from build123d import *
from build123d.topology import SkipClean

# Parameters (mm, degrees)
ESQUISSE2_R                                      = 31.5
ESQUISSE2_W                                      = 32
ESQUISSE2_H                                      = 32
BOSS_EXTRU_1_DEPTH                               = 3
BOSS_EXTRU_2_START                               = -100
ESQUISSE4_R                                      = 35
ESQUISSE4_R_2                                    = 31.5
BOSS_EXTRU_2_DEPTH                               = 100
BOSS_EXTRU_3_OUTLINE_R                           = 31.5
BOSS_EXTRU_3_OUTLINE_W                           = 43
BOSS_EXTRU_3_OUTLINE_H                           = 42.5
BOSS_EXTRU_3_DEPTH                               = 97
ESQUISSE6_R                                      = 31.5
ENL_V_MAT_EXTRU_1_DEPTH                          = 10
ESQUISSE7_R                                      = 49
ESQUISSE7_R_2                                    = 35
BOSS_EXTRU_4_DEPTH                               = 10
BOSS_EXTRU_5_START                               = 30
BOSS_EXTRU_5_DEPTH                               = 30
BOSS_EXTRU_6_START                               = 16
BOSS_EXTRU_6_DEPTH                               = 16
CONG_1_R                                         = 10
ESQUISSE11_W                                     = 137.068824
ESQUISSE11_H                                     = 50.889867
ENL_V_MAT_EXTRU_2_DEPTH                          = 153
CHAMBRAGE_POUR_VIS_T_TE_RONDE_6_PANS_D           = 5.3
CHAMBRAGE_POUR_VIS_T_TE_RONDE_6_PANS_DEPTH       = 18
CHAMBRAGE_POUR_VIS_T_TE_RONDE_6_PANS_CBORE_D     = 10.5
CHAMBRAGE_POUR_VIS_T_TE_RONDE_6_PANS_CBORE_DEPTH = 2.75
CHAMBRAGE_POUR_VIS_T_TE_RONDE_6_PANS_TIP         = 1.592281
ESQUISSE18_R                                     = 2.6
ENL_V_MAT_EXTRU_4_DEPTH                          = 25
ESQUISSE19_R                                     = 4.6
ENL_V_MAT_EXTRU_5_DEPTH                          = 25
ESQUISSE20_W                                     = 2
ESQUISSE20_H                                     = 3
ENL_V_MAT_EXTRU_6_DEPTH                          = 45
ENL_V_START                                      = -90
ENL_V_MAT_EXTRU_7_DEPTH                          = 90


# Read off the part's stored shape, not the designer's step: Boss.-Extru.3
with BuildPart() as part:
    # Esquisse2 → Boss.-Extru.1 (new body)
    with BuildSketch(Plane.XY):
        Circle(ESQUISSE2_R)
        with Locations((0.409228, -1.432297)):
            Rectangle(ESQUISSE2_W, ESQUISSE2_H, mode=Mode.SUBTRACT)
    extrude(amount=BOSS_EXTRU_1_DEPTH)

    # Esquisse4 → Boss.-Extru.2 (add)
    with BuildSketch(Plane.XY.offset(3).offset(BOSS_EXTRU_2_START)):
        Circle(ESQUISSE4_R)
        Circle(ESQUISSE4_R_2, mode=Mode.SUBTRACT)
    extrude(amount=BOSS_EXTRU_2_DEPTH)

    # Boss.-Extru.3 outline → Boss.-Extru.3 (add)
    with BuildSketch(Plane(origin=(0, 0, 0), x_dir=(-1, 0, 0), z_dir=(0, 0, -1))):
        Circle(BOSS_EXTRU_3_OUTLINE_R)
        with Locations((-0.409228, -1.182297)):
            Rectangle(BOSS_EXTRU_3_OUTLINE_W, BOSS_EXTRU_3_OUTLINE_H, mode=Mode.SUBTRACT)
    extrude(amount=BOSS_EXTRU_3_DEPTH)

    # Esquisse6 → Enlèv. mat.-Extru.1 (cut)
    with BuildSketch(Plane(origin=(0, 0, -97), x_dir=(-1, 0, 0), z_dir=(0, 0, -1))):
        Circle(ESQUISSE6_R)
    extrude(amount=-ENL_V_MAT_EXTRU_1_DEPTH, mode=Mode.SUBTRACT)

    # Esquisse7 → Boss.-Extru.4 (add)
    with BuildSketch(Plane(origin=(0, 0, -97), x_dir=(-1, 0, 0), z_dir=(0, 0, -1))):
        Circle(ESQUISSE7_R)
        with Locations(Location((0, 0, 0), (0, 0, 180))):
            Circle(ESQUISSE7_R_2, mode=Mode.SUBTRACT)
    extrude(amount=-BOSS_EXTRU_4_DEPTH)

    # Esquisse8 → Boss.-Extru.5 (add)
    with SkipClean():  # the faces are left unmerged after this step: merging them gives an invalid solid
        with BuildSketch(Plane(origin=(0, 0, -97), x_dir=(-1, 0, 0), z_dir=(0, 0, -1)).offset(BOSS_EXTRU_5_START)):
            with BuildLine():
                Line((-47.96874, 10), (-29.870554, 10))
                ThreePointArc((-29.870554, 10), (-31.5, 0), (-29.870554, -10))
                Line((-29.870554, -10), (-47.96874, -10))
                ThreePointArc((-47.96874, -10), (-49, 0), (-47.96874, 10))
            make_face()
            with BuildLine():
                Line((29.870554, 10), (47.96874, 10))
                ThreePointArc((47.96874, 10), (49, 0), (47.96874, -10))
                Line((47.96874, -10), (29.870554, -10))
                ThreePointArc((29.870554, -10), (31.5, 0), (29.870554, 10))
            make_face()
        extrude(amount=-BOSS_EXTRU_5_DEPTH)

    # Esquisse10 → Boss.-Extru.6 (add)
    with SkipClean():  # the faces are left unmerged after this step: merging them gives an invalid solid
        with BuildSketch(Plane(origin=(0, 0, -127), x_dir=(-1, 0, 0), z_dir=(0, 0, -1)).offset(BOSS_EXTRU_6_START)):
            with BuildLine():
                Line((47.96874, 10), (-47.96874, 10))
                ThreePointArc((-47.96874, 10), (-49, 0), (-47.96874, -10))
                Line((-47.96874, -10), (47.96874, -10))
                ThreePointArc((47.96874, -10), (49, 0), (47.96874, 10))
            make_face()
        extrude(amount=-BOSS_EXTRU_6_DEPTH)

    # Congé1
    cong_1_edges = [part.edges().sort_by_distance(p)[0] for p in [
        (-49, 0, -143),
        (49, 0, -143),
    ]]
    fillet(cong_1_edges, radius=CONG_1_R)

    # Esquisse11 → Enlèv. mat.-Extru.2 (cut)
    with SkipClean():  # the faces are left unmerged after this step: merging them gives an invalid solid
        with BuildSketch(Plane(origin=(0, 0, -143), x_dir=(-1, 0, 0), z_dir=(0, 0, -1))):
            with Locations((0, -25.444933)):
                Rectangle(ESQUISSE11_W, ESQUISSE11_H)
        extrude(amount=-ENL_V_MAT_EXTRU_2_DEPTH, mode=Mode.SUBTRACT)

    # Chambrage pour Vis à tête ronde à 6 pans creux M51
    with Locations(Plane(origin=(0, 10, 0), x_dir=(1, 0, 0), z_dir=(0, 1, 0))):
        with Locations((-38.919647, 112), (38.919647, 112), (0, 135)):
            CounterBoreHole(CHAMBRAGE_POUR_VIS_T_TE_RONDE_6_PANS_D / 2, CHAMBRAGE_POUR_VIS_T_TE_RONDE_6_PANS_CBORE_D / 2, CHAMBRAGE_POUR_VIS_T_TE_RONDE_6_PANS_CBORE_DEPTH, depth=CHAMBRAGE_POUR_VIS_T_TE_RONDE_6_PANS_DEPTH)
            with Locations((0, 0, -(CHAMBRAGE_POUR_VIS_T_TE_RONDE_6_PANS_DEPTH + CHAMBRAGE_POUR_VIS_T_TE_RONDE_6_PANS_TIP / 2))):  # 118° drill point
                Cone(0, CHAMBRAGE_POUR_VIS_T_TE_RONDE_6_PANS_D / 2, CHAMBRAGE_POUR_VIS_T_TE_RONDE_6_PANS_TIP, mode=Mode.SUBTRACT)

    # Esquisse18 → Enlèv. mat.-Extru.4 (cut, symmetric)
    with SkipClean():  # the faces are left unmerged after this step: merging them gives an invalid solid
        with BuildSketch(Plane(origin=(0, 15, 0), x_dir=(-1, 0, 0), z_dir=(0, -1, 0))):
            with Locations(Location((28, 12, 0), (0, 0, 90))):
                Circle(ESQUISSE18_R)
            with Locations(Location((-28, 12, 0), (0, 0, 90))):
                Circle(ESQUISSE18_R)
            with Locations(Location((28, 72, 0), (0, 0, 90))):
                Circle(ESQUISSE18_R)
            with Locations(Location((-28, 72, 0), (0, 0, 90))):
                Circle(ESQUISSE18_R)
        extrude(amount=ENL_V_MAT_EXTRU_4_DEPTH, both=True, mode=Mode.SUBTRACT)

    # Esquisse19 → Enlèv. mat.-Extru.5 (cut)
    with SkipClean():  # the faces are left unmerged after this step: merging them gives an invalid solid
        with BuildSketch(Plane.ZX.offset(35)):
            with Locations((-72, 28)):
                Circle(ESQUISSE19_R)
            with Locations((-12, 28)):
                Circle(ESQUISSE19_R)
            with Locations((-12, -28)):
                Circle(ESQUISSE19_R)
            with Locations((-72, -28)):
                Circle(ESQUISSE19_R)
        extrude(amount=-ENL_V_MAT_EXTRU_5_DEPTH, mode=Mode.SUBTRACT)

    # Esquisse20 → Enlèv. mat.-Extru.6 (cut)
    with SkipClean():  # the faces are left unmerged after this step: merging them gives an invalid solid
        with BuildSketch(Plane(origin=(0, 0, -87), x_dir=(-1, 0, 0), z_dir=(0, 0, -1))):
            with Locations((22.090772, 1.5)):
                Rectangle(ESQUISSE20_W, ESQUISSE20_H)
        extrude(amount=-ENL_V_MAT_EXTRU_6_DEPTH, mode=Mode.SUBTRACT)

    # Esquisse21 → Enlèv. mat.-Extru.7 (cut)
    with SkipClean():  # the faces are left unmerged after this step: merging them gives an invalid solid
        with BuildSketch(Plane.XY.offset(3).offset(ENL_V_START)):
            with BuildLine():
                Line((-35, 0), (-34, 0))
                ThreePointArc((-34, 0), (0, 34), (34, 0))
                Line((34, 0), (35, 0))
                ThreePointArc((35, 0), (0, 35), (-35, 0))
            make_face()
        extrude(amount=ENL_V_MAT_EXTRU_7_DEPTH, mode=Mode.SUBTRACT)


solid = part.part
Can you work these out from the model? Positions are in its coordinate system, mm. A direction names the side the tool comes from. Give positions to 0.01 mm unless a question says otherwise; leave off trailing zeros. Loops run counter-clockwise (first coordinate to the right, second up) from the corner with the lowest first, then second, coordinate; pieces in that order, holes last. Notation, with made-up numbers: (-16.75, 39) - (-5.75, 39) arc R22 cw to (-5.75, 65) - close; hole circle Ø8 at (40.5, 23.25). An arc over 180 degrees is marked (long way). Answer as a JSON object with one key per item and string values.
Q1. If I drill on L1, parallel to Z at x = 28, y = 18; L2, parallel to Z at x = -28, y = 5; L3, parallel to X at y = 7, z = -12, over which ranges is the centre line in solid material (lowest first)?
Geometry says:
{"L1": "-97 to -76.6, -67.4 to -16.6, -7.4 to 3", "L2": "-143 to -127, -87 to -74.6, -69.4 to -14.6, -9.4 to 3", "L3": "-33.27 to -30.6, -25.4 to -21.09, 21.91 to 25.4, 30.6 to 33.27"}
Q2. Imagine slicing it at D-D on z = -85.5. Write out the boundary of the cut face in (x, y), plus the area to 3 significant figures.
Geometry says:
{"outline": "(-34, 0) - (-23.09, 0) - (-23.09, 3) - (-21.09, 3) - (-21.09, 20.07) - (21.91, 20.07) - (21.91, 0) - (34, 0) arc R34 ccw to start", "area": "947 mm²"}
Q3. Imagine slicing it at B-B on z = -112. Write out the boundary of the cut face in (x, y).
Geometry says:
{"outline": "(-49, 0) - (-41.57, 0) - (-41.57, 7.25) - (-44.17, 7.25) - (-44.17, 10) - (-47.97, 10) arc R49 ccw to start; (-36.27, 0) - (-31.5, 0) arc R31.5 cw to (-29.87, 10) - (-33.67, 10) - (-33.67, 7.25) - (-36.27, 7.25) - close; (29.87, 10) arc R31.5 cw to (31.5, 0) - (36.27, 0) - (36.27, 7.25) - (33.67, 7.25) - (33.67, 10) - close; (41.57, 0) - (49, 0) arc R49 ccw to (47.97, 10) - (44.17, 10) - (44.17, 7.25) - (41.57, 7.25) - close"}
Q4. Will these pins go through, and if not, where does the flat tip stop? P1, Ø10, axis at x = 20.5, y = 24, coming from the -Z side; P2, Ø2, axis at x = -21.5, z = -54, coming from the -Y side; P3, Ø5.5, axis at x = 28, z = -12, coming from the +Y side; P4, Ø3, axis at x = 28, z = -12, coming from the +Y side.
Geometry says:
{"P1": "z = -97", "P2": "y = 3", "P3": "y = 10", "P4": "through"}
Q5. If we mould it in two halves opening along Z, with no side actions, what happens to faces 5 (the cylindrical face through (28.78, 5.07, -14.48)), 6 (the flat face through (0, 17, 3)), 7 (the flat face through (0, 5, -127)), 8 (the flat face through (16.409, 7, 1))? For each: pulls with the +Z half, pulls with the -Z half, needs draft (parallel to the pull), parting line crosses it, or undercut.
Geometry says:
{"face 5": "undercut", "face 6": "pulls with the +Z half", "face 7": "undercut", "face 8": "needs draft"}
Q6. Imagine slicing it at A-A on x = 0. Write out the boundary of the cut face in (y, z).
Geometry says:
{"outline": "(0, -143) - (10, -143) - (10, -140.25) - (7.25, -140.25) - (7.25, -137.65) - (0, -137.65) - close; (0, -132.35) - (7.25, -132.35) - (7.25, -129.75) - (10, -129.75) - (10, -127) - (0, -127) - close; (14.57, 0) - (20.07, 0) - (20.07, -87) - (31.5, -87) - (31.5, -97) - (49, -97) - (49, -87) - (34, -87) - (34, 3) - (14.57, 3) - close"}
Q7. Which directions (+Z, -Z, +X, -X, +Y, -Y) give clear straight access to the entire face, cutting with the end or side of a thin tool? Please do faces 1 (the flat face through (1, 20.068, -43)), 2 (the cylindrical face through (-39.603, 8.644, -117.205)), 3 (the flat face through (-21.091, 10, -43)), 4 (the flat face through (1, 34, -97)).
Geometry says:
{"face 1": "-Z, -Y", "face 2": "+Y", "face 3": "-Y", "face 4": "-Z, +X, -X, +Y"}
Q8. Imagine slicing it at C-C on y = 12. Write out the boundary of the cut face in (x, z).
Geometry says:
{"outline": "(-47.51, -97) - (-29.12, -97) - (-29.12, -87) - (-21.09, -87) - (-21.09, 0) - (-15.59, 0) - (-15.59, 3) - (-31.81, 3) - (-31.81, -9.43) arc R4.6 cw (long way) to (-31.81, -14.57) - (-31.81, -69.43) arc R4.6 cw (long way) to (-31.81, -74.57) - (-31.81, -87) - (-47.51, -87) - close; (16.41, 0) - (21.91, 0) - (21.91, -87) - (29.12, -87) - (29.12, -97) - (47.51, -97) - (47.51, -87) - (31.81, -87) - (31.81, -74.57) arc R4.6 cw (long way) to (31.81, -69.43) - (31.81, -14.57) arc R4.6 cw (long way) to (31.81, -9.43) - (31.81, 3) - (16.41, 3) - close"}
